Answer from the drawing. Dimensions are ordinates in mm from the lowest x, y and z of the part. Round coordinates to 2 decimals unless told otherwise and drop trailing zeros. Order: outer loops, then holes, each group sorted by start corner. A loop starts at its lowest first (then second) coordinate and runs counter-clockwise, first axis right, second up. Notation, with made-up numbers: M 42.25,-22 L 74.25,-22 A16 cw 74.25,-3 Z; hole C 38,21 d6. An arc over 180 degrees is marked long. Write item = value, one per line. Start each with the question number.
(1) A cutting plane is placed at D-D, the plane y = 37. Determine the outline of the cut face in (x, z), and give its area (3 significant figures).
(2) A cutting plane is placed at A-A, the plane x = 21. Determine the outline of the cut face in (y, z), and give its area (3 significant figures).
(3) A cutting plane is placed at C-C, the plane z = 3.3. Determine the outline of the cut face in (x, y), and give its area (3 significant figures).
(4) This flat-tipped pin is pushed along its axis until it touches: pin 1 (2 mm diameter, centred on y = 29.5, z = 1.5, fed in from +X). Where does it stop, or does it pass through?
(5) Straight lines are drawn through the part: probe 1 along Y at (x, z) = (21, 1.55); probe 2 along Y at (x, z) = (20, 2.6); probe 3 along Y at (x, z) = (17, 1.65). For each, find the intervals that lie inside material, in ascending order. Write a range as from..to.
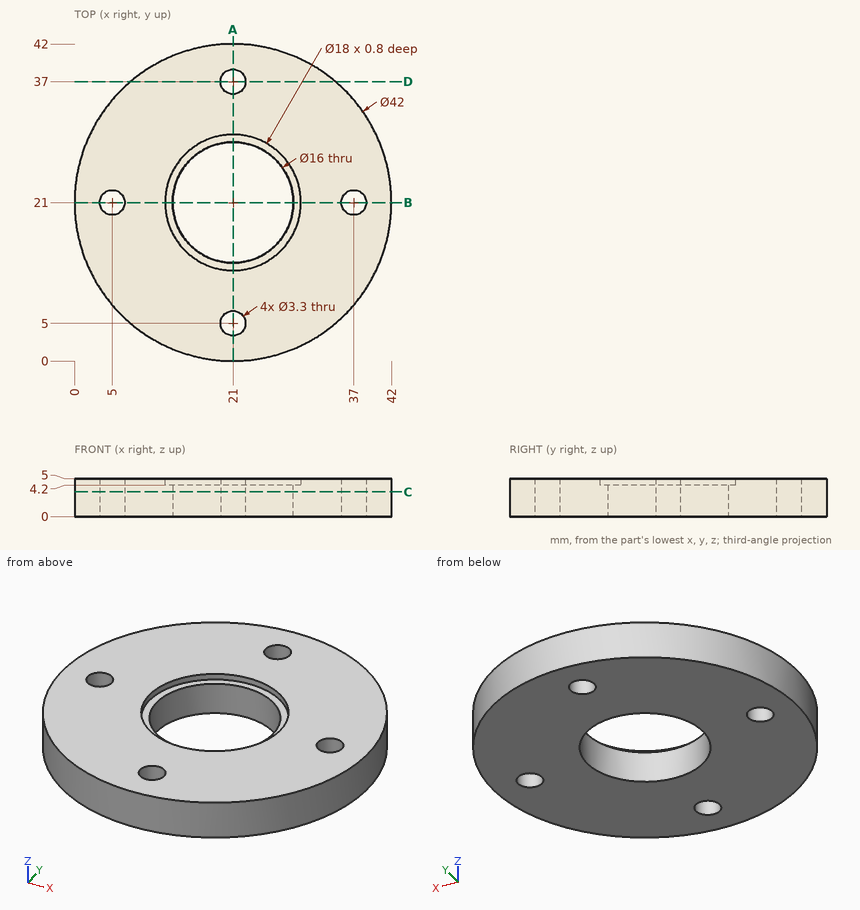
Reported:
q1.outline = M 7.4,0 L 19.35,0 L 19.35,5 L 7.4,5 Z; M 22.65,0 L 34.6,0 L 34.6,5 L 22.65,5 Z
q1.area = 120 mm²
q2.outline = M 0,0 L 3.35,0 L 3.35,5 L 0,5 Z; M 6.65,0 L 13,0 L 13,4.2 L 12,4.2 L 12,5 L 6.65,5 Z; M 29,0 L 35.35,0 L 35.35,5 L 30,5 L 30,4.2 L 29,4.2 Z; M 38.65,0 L 42,0 L 42,5 L 38.65,5 Z
q2.area = 95.4 mm²
q3.outline = C 21,21 d42; hole C 5,21 d3.3; hole C 21,21 d16; hole C 21,5 d3.3; hole C 21,37 d3.3; hole C 37,21 d3.3
q3.area = 1,150 mm²
q4.pin_1 = 40.62
q5.probe_1 = 0..3.35, 6.65..13, 29..35.35, 38.65..42
q5.probe_2 = 0.02..3.69, 6.31..13.06, 28.94..35.69, 38.31..41.98
q5.probe_3 = 0.38..14.07, 27.93..41.62
